from build123d import *

# Parameters (mm, degrees)
SKIZZE6_R                            = 1.05
SCHNITT_LINEAR_AUSTRAGEN3_DEPTH      = 46
SKIZZE7_R                            = 2.75
SCHNITT_LINEAR_AUSTRAGEN4_DEPTH      = 2.5
AUFSATZ_LINEAR_START                 = -2
AUFSATZ_LINEAR_AUSTRAGEN6_DEPTH      = 6
AUFSATZ_LINEAR_AUSTRAGEN7_DEPTH      = 4.5
SKIZZE14_R                           = 1.15
SCHNITT_LINEAR_AUSTRAGEN5_DEPTH      = 7.5
SKIZZE17_W                           = 6.5
SKIZZE17_H                           = 2.4
SCHNITT_LINEAR_AUSTRAGEN9_DEPTH      = 18
SCHNITT_LINEAR_AUSTRAGEN9_DEPTH_BACK = 18
SCHNITT_LINEAR_START                 = -3.300852
SKIZZE18_W                           = 12.760877712
SKIZZE18_H                           = 6.5
SCHNITT_LINEAR_AUSTRAGEN10_DEPTH     = 3.300852
SKIZZE19_R                           = 3.75
SCHNITT_LINEAR_AUSTRAGEN11_DEPTH     = 6


with BuildPart() as part:
    # Skizze5 → Rotation1 (revolve)
    with BuildSketch(Plane(origin=(0, 0, 0), x_dir=(0, 0, -1), z_dir=(1, 0, 0))):
        Polygon((40, 7.75), (0, 7.75), (0, 3.75), (-1, 3.75), (-1, 3.25), (-2.6, 3.25), (-2.6, 2), (-5, 2), (-5, 10), (40, 10), align=None)
    revolve(axis=Axis((0, 0, 0), (0, 0, 1)))

    # Skizze6 → Schnitt-Linear austragen3 (cut, through all)
    with BuildSketch(Plane.XY.offset(5)):
        with Locations((0, 5.5)):
            Circle(SKIZZE6_R)
        with Locations((0, -5.5)):
            Circle(SKIZZE6_R)
        with Locations((5.5, 0)):
            Circle(SKIZZE6_R)
        with Locations((-5.5, 0)):
            Circle(SKIZZE6_R)
    extrude(amount=-SCHNITT_LINEAR_AUSTRAGEN3_DEPTH, mode=Mode.SUBTRACT)

    # Skizze7 → Schnitt-Linear austragen4 (cut)
    with BuildSketch(Plane.XY.offset(5)):
        with Locations((0, 5.5)):
            Circle(SKIZZE7_R)
        with Locations((0, -5.5)):
            Circle(SKIZZE7_R)
        with Locations((5.5, 0)):
            Circle(SKIZZE7_R)
        with Locations((-5.5, 0)):
            Circle(SKIZZE7_R)
    extrude(amount=-SCHNITT_LINEAR_AUSTRAGEN4_DEPTH, mode=Mode.SUBTRACT)

    # Skizze12 → Aufsatz-Linear austragen6 (add)
    with BuildSketch(Plane.XY.offset(5).offset(AUFSATZ_LINEAR_START)):
        with BuildLine():
            Line((-10, 0), (-10, 8))
            Line((-10, 8), (-6, 8))
            ThreePointArc((-6, 8), (-8.94427191, 4.472135955), (-10, 0))
        make_face()
        with BuildLine():
            Line((10, 8), (6, 8))
            ThreePointArc((6, 8), (8.94427191, 4.472135955), (10, 0))
            Line((10, 0), (10, 8))
        make_face()
    aufsatz_linear_austragen6 = extrude(amount=-AUFSATZ_LINEAR_AUSTRAGEN6_DEPTH)

    # Spiegeln1: Aufsatz-Linear austragen6 across plane
    add(aufsatz_linear_austragen6.mirror(Plane(origin=(0, 0, -18.5), x_dir=(1, 0, 0), z_dir=(0, 0, -1))))

    # Skizze13 → Aufsatz-Linear austragen7 (add)
    with BuildSketch(Plane(origin=(0, 8, 0), x_dir=(1, 0, 0), z_dir=(0, 1, 0))):
        with BuildLine():
            Line((-14, 40), (-10, 40))
            Line((-10, 40), (-10, 34))
            Line((-10, 34), (-14, 34))
            ThreePointArc((-14, 34), (-17, 37), (-14, 40))
        make_face()
        with BuildLine():
            Line((14, 34), (10, 34))
            Line((10, 34), (10, 40))
            Line((10, 40), (14, 40))
            ThreePointArc((14, 40), (17, 37), (14, 34))
        make_face()
        with BuildLine():
            Line((14, -3), (10, -3))
            Line((10, -3), (10, 3))
            Line((10, 3), (14, 3))
            ThreePointArc((14, 3), (17, 0), (14, -3))
        make_face()
        with BuildLine():
            Line((-14, 3), (-10, 3))
            Line((-10, 3), (-10, -3))
            Line((-10, -3), (-14, -3))
            ThreePointArc((-14, -3), (-17, 0), (-14, 3))
        make_face()
    extrude(amount=-AUFSATZ_LINEAR_AUSTRAGEN7_DEPTH)

    # Skizze14 → Schnitt-Linear austragen5 (cut, through all)
    with BuildSketch(Plane(origin=(0, 3.5, 0), x_dir=(-1, 0, 0), z_dir=(0, -1, 0))):
        with Locations((14, 0)):
            Circle(SKIZZE14_R)
        with Locations((-14, 0)):
            Circle(SKIZZE14_R)
        with Locations((-14, 37)):
            Circle(SKIZZE14_R)
        with Locations((14, 37)):
            Circle(SKIZZE14_R)
    extrude(amount=-SCHNITT_LINEAR_AUSTRAGEN5_DEPTH, mode=Mode.SUBTRACT)

    # Skizze17 → Schnitt-Linear austragen9 (cut, two sides)
    with BuildSketch(Plane(origin=(0, 0, 0), x_dir=(0, 0, -1), z_dir=(1, 0, 0))) as schnitt_linear_austragen9_sk:
        with Locations((10.75, 8.9)):
            Rectangle(SKIZZE17_W, SKIZZE17_H)
        with Locations((26.25, 8.9)):
            Rectangle(SKIZZE17_W, SKIZZE17_H)
    extrude(amount=SCHNITT_LINEAR_AUSTRAGEN9_DEPTH, mode=Mode.SUBTRACT)
    extrude(schnitt_linear_austragen9_sk.sketch, amount=-SCHNITT_LINEAR_AUSTRAGEN9_DEPTH_BACK, mode=Mode.SUBTRACT)

    # Skizze18 → Schnitt-Linear austragen10 (cut)
    with BuildSketch(Plane(origin=(0, 7.7, 0), x_dir=(1, 0, 0), z_dir=(0, 1, 0)).offset(SCHNITT_LINEAR_START)):
        with Locations((0, 10.75)):
            Rectangle(SKIZZE18_W, SKIZZE18_H)
        with Locations((0, 26.25)):
            Rectangle(SKIZZE18_W, SKIZZE18_H)
    extrude(amount=SCHNITT_LINEAR_AUSTRAGEN10_DEPTH, mode=Mode.SUBTRACT)

    # Skizze19 → Schnitt-Linear austragen11 (cut, through all)
    with BuildSketch(Plane(origin=(0, 0, 0), x_dir=(-1, 0, 0), z_dir=(0, 0, -1))):
        Circle(SKIZZE19_R)
    extrude(amount=-SCHNITT_LINEAR_AUSTRAGEN11_DEPTH, mode=Mode.SUBTRACT)


solid = part.part
Could you check a few things on this model? Use its own coordinates, in mm. A direction names the side the tool comes from. Give positions to 0.01 mm unless a question says otherwise; leave off trailing zeros. Write each loop counter-clockwise with the first axis right and the second up, starting at its lowest first coordinate (ties: lowest second). Pieces come first, ordered by that corner, then holes. Notation, with made-up numbers: (20, -14) -> (36, -14) arc R23 cw to (36, 5) -> close; hole circle Ø2 at (71, 78). An arc over 180 degrees is marked (long way). Answer as a JSON object with one key per item and string values.
Q1. Which directions (+Z, -Z, +X, -X, +Y, -Y) give clear straight access to the entire face, cutting with the end or side of a thin tool? Please do faces 1 (the flat face through (11, 6, 3)), 2 (the flat face through (-11, 6, -3)), 3 (the flat face through (-6.38, 6, -11)).
Taken from the geometry:
{"face 1": "+Z, +X, +Y", "face 2": "-X, +Y", "face 3": "+Y"}
Q2. Suppose I cut it at A-A on z = -37. Write out the boundary of the cut face in (x, y).
Taken from the geometry:
{"outline": "(-17, 3.5) -> (-15.15, 3.5) -> (-15.15, 8) -> (-17, 8) -> close; (-12.85, 3.5) -> (-10, 3.5) -> (-10, 0) arc R10 ccw to (10, 0) -> (10, 3.5) -> (12.85, 3.5) -> (12.85, 8) -> (6, 8) arc R10 ccw to (-6, 8) -> (-12.85, 8) -> close; (15.15, 3.5) -> (17, 3.5) -> (17, 8) -> (15.15, 8) -> close; hole circle Ø15.5 at (0, 0)"}
Q3. We'd pull the mould along Y, two halves only. Please class faces 4 (the flat face through (7, 0, 2.5)), 5 (the flat face through (13, 3.5, -1)), 6 (the flat face through (10, 2, -37)): released by +Y, released by -Y, zero draft, split by the parting line, or undercut.
Taken from the geometry:
{"face 4": "undercut", "face 5": "released by -Y", "face 6": "zero draft"}
Q4. Please list where these lines run through material, in increasing order: L1, parallel to Z at x = -14, y = 6.35; L2, parallel to Y at x = 0, z = 1; L3, parallel to Z at x = 15, y = 4.5.
Taken from the geometry:
{"L1": "z = -40 to -38.15, -35.85 to -34, -3 to -1.15, 1.15 to 3", "L2": "y = -10 to -6.55, -4.45 to -3.75, 3.75 to 4.45, 6.55 to 10", "L3": "z = -39.83 to -37.57, -36.43 to -34.17, -2.83 to -0.57, 0.57 to 2.83"}
Q5. Suppose I cut it at D-D on z = -4. Write out the boundary of the cut face in (x, y), then the cut area to 3 significant figures.
Taken from the geometry:
{"outline": "circle Ø20 at (0, 0); hole circle Ø15.5 at (0, 0)", "area": "125 mm²"}
Q6. Suppose I cut it at C-C on y = -6. Write out the boundary of the cut face in (x, z), then the cut area to 3 significant figures.
Taken from the geometry:
{"outline": "(-8, -40) -> (-4.91, -40) -> (-4.91, 0) -> (-0.92, 0) -> (-0.92, 2.5) -> (-2.7, 2.5) -> (-2.7, 5) -> (-8, 5) -> close; (0.92, 0) -> (4.91, 0) -> (4.91, -40) -> (8, -40) -> (8, 5) -> (2.7, 5) -> (2.7, 2.5) -> (0.92, 2.5) -> close", "area": "309 mm²"}
Q7. Will these pins go through, and if not, where does the flat tip stop? pin 1 Ø10 at (x, y) = (3, -1.5) entering from -Z; pin 2 Ø3 at (y, z) = (1.5, 0.5) entering from +X; pin 3 Ø2 at (x, y) = (-4.5, -1) entering from -Z; pin 4 Ø6 at (y, z) = (-4.5, -11) entering from +X.
Taken from the geometry:
{"pin 1": "stops at z = -40", "pin 2": "stops at x = 10", "pin 3": "stops at z = 0", "pin 4": "stops at x = 9.89"}
Q8. Suppose I cut it at B-B on x = -5.5. Write out the boundary of the cut face in (y, z), then the cut area to 3 significant figures.
Taken from the geometry:
{"outline": "(-8.35, -40) -> (-5.46, -40) -> (-5.46, 0) -> (-1.05, 0) -> (-1.05, 2.5) -> (-2.75, 2.5) -> (-2.75, 5) -> (-8.35, 5) -> close; (1.05, 0) -> (5.46, 0) -> (5.46, -7.5) -> (8.35, -7.5) -> (8.35, 5) -> (2.75, 5) -> (2.75, 2.5) -> (1.05, 2.5) -> close; (5.46, -40) -> (8.35, -40) -> (8.35, -29.5) -> (5.46, -29.5) -> close; (5.46, -23) -> (8.35, -23) -> (8.35, -14) -> (5.46, -14) -> close", "area": "258 mm²"}
